```python
from build123d import *

# Parameters (mm, degrees)
F0_W     = 140
F0_H     = 60
F1_DEPTH = 60
F2_R     = 10
F5_DEPTH = 10
F3_R     = 10
F6_DEPTH = 10
F4_R     = 10
F7_DEPTH = 79.5
F8_R     = 5


with BuildPart() as f1:
    # F0 (on Top) → F1 (new body)
    with BuildSketch(Plane.XY):
        Rectangle(F0_W, F0_H)
    extrude(amount=F1_DEPTH)

    # F2 (on face) → F5 (join)
    with BuildSketch(Plane.XY.offset(60)):
        with Locations((-40, 0)):
            Circle(F2_R)
    extrude(amount=F5_DEPTH)

    # F3 (on face) → F6 (cut)
    with BuildSketch(Plane.XY.offset(60)):
        with Locations((40, 0)):
            Circle(F3_R)
    extrude(amount=-F6_DEPTH, mode=Mode.SUBTRACT)

    # F4 (on face) → F7 (cut)
    with BuildSketch(Plane.XY.offset(60)):
        Circle(F4_R)
    extrude(amount=-F7_DEPTH, mode=Mode.SUBTRACT)

    # F8
    f8_edges = [f1.edges().sort_by_distance(p)[0] for p in [
        (-70, 0, 60),
        (0, -30, 60),
        (70, 0, 60),
        (0, 30, 60),
        (-50, 0, 60),
        (-10, 0, 60),
        (30, 0, 60),
    ]]
    fillet(f8_edges, radius=F8_R)


solid = f1.part
```
Could you check a few things on this model? Use its own coordinates, in mm. A direction names the side the tool comes from. Round coordinates to 2 decimals unless told otherwise and drop trailing zeros. Loops run counter-clockwise (first coordinate to the right, second up) from the corner with the lowest first, then second, coordinate; pieces in that order, holes last. Notation, with made-up numbers: (-20, 49.5) - (12, 49.5) arc R36 ccw to (12, 88.5) - close; hole circle Ø11 at (21, 86). An arc over 180 degrees is marked (long way). Answer in a Markdown table with one row per item. Add a question column.
(1) For faces 1 (the face through (40, 0, 50)), 2 (the face through (-70, 0, 27)), which set-ups out of +Z, -Z, +X, -X, +Y, -Y let a thin tool reach every point of the face, with its end or its side?
(2) If we section it at B-B (x = 0): Please give me the cut outline in (y, z).
(3) If we section it at A-A (y = 0): Please give me the cut outline in (x, z).
(4) If we mould it in two halves opening along Y, with no side actions, what happens to faces 3 (the face through (70, 0, 27)), 4 (the face through (-1, 30, 27)), 5 (the face through (30, 0, 53)), 6 (the face through (-50, 0, 67))? For each: pulls with the +Y half, pulls with the -Y half, needs draft (parallel to the pull), parting line crosses it, or undercut.
(5) I'm going to push flat-ended pins straight in: pin 1 (8 mm diameter, centred on x = 31, y = -12, fed in from -Z); pin 2 (12 mm diameter, centred on x = 0, y = 0, fed in from +Z); pin 3 (10 mm diameter, centred on x = 37.5, y = 4, fed in from +Z); pin 4 (2 mm diameter, centred on x = -28.5, y = 15, fed in from +Z). Where does each tip first touch, or does it pass through?
(6) If we section it at D-D (x = 40): Please give me the cut outline in (y, z), plus the area to 3 significant figures.
(7) If we section it at C-C (z = 29): Please give me the cut outline in (x, y), plus the area to 3 significant figures.
(8) I need wall thicknesses on line 1 along Y through (x, z) = (40, 52.8); line 2 along Z through (x, y) = (-24.5, 16); line 3 along X through (y, z) = (3.5, 10.5). Which ranges of each line are inside material? Lowest first, please.
Model answer:
| question | item | result |
|---|---|---|
| 1 | face 1 | +Z |
| 1 | face 2 | +Z, -Z, -X, +Y, -Y |
| 2 | outline | (-30, 0) - (-10, 0) - (-10, 55) arc R5 ccw to (-15, 60) - (-25, 60) arc R5 ccw to (-30, 55) - close; (10, 0) - (30, 0) - (30, 55) arc R5 ccw to (25, 60) - (15, 60) arc R5 ccw to (10, 55) - close |
| 3 | outline | (-70, 0) - (-10, 0) - (-10, 55) arc R5 ccw to (-15, 60) - (-25, 60) arc R5 cw to (-30, 65) - (-30, 70) - (-50, 70) - (-50, 65) arc R5 cw to (-55, 60) - (-65, 60) arc R5 ccw to (-70, 55) - close; (10, 0) - (70, 0) - (70, 55) arc R5 ccw to (65, 60) - (55, 60) arc R5 ccw to (50, 55) - (50, 50) - (30, 50) - (30, 55) arc R5 ccw to (25, 60) - (15, 60) arc R5 ccw to (10, 55) - close |
| 4 | face 3 | needs draft |
| 4 | face 4 | pulls with the +Y half |
| 4 | face 5 | undercut |
| 4 | face 6 | parting line crosses it |
| 5 | pin 1 | stops at z = 0 |
| 5 | pin 2 | passes through |
| 5 | pin 3 | stops at z = 50 |
| 5 | pin 4 | stops at z = 60 |
| 6 | outline | (-30, 0) - (30, 0) - (30, 55) arc R5 ccw to (25, 60) - (15, 60) arc R5 ccw to (10, 55) - (10, 50) - (-10, 50) - (-10, 55) arc R5 ccw to (-15, 60) - (-25, 60) arc R5 ccw to (-30, 55) - close |
| 6 | area | 3,380 mm² |
| 7 | outline | (-70, -30) - (70, -30) - (70, 30) - (-70, 30) - close; hole circle Ø20 at (0, 0) |
| 7 | area | 8,090 mm² |
| 8 | line 1 | y = -30 to -10, 10 to 30 |
| 8 | line 2 | z = 0 to 60 |
| 8 | line 3 | x = -70 to -9.37, 9.37 to 70 |
